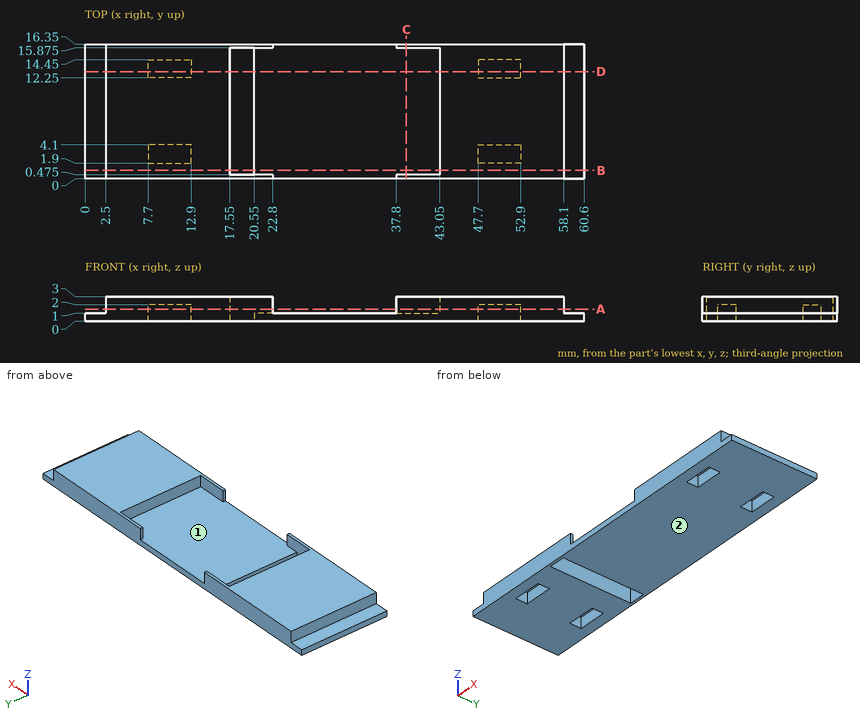
Part print with two shaded views. Sizes in mm from the minimum x, y, z corner. Round coordinates to 2 decimals unless told otherwise and drop trailing zeros. Order: outer loops, then holes, each group sorted by start corner. A loop starts at its lowest first (then second) coordinate and runs counter-clockwise, first axis right, second up. Notation, with made-up numbers: (9, 24) -> (29, 24) arc R16 ccw to (29, 53) -> close; hole circle Ø1 at (36, -22.5). An arc over 180 degrees is marked (long way). Use one line per item in the form item = value.
Item 1: Cut at B-B, the plane y = 1. Write the cut outline in (x, z), and give its area (3 significant figures).
Returned:
outline = (0, 0) -> (17.55, 0) -> (17.55, 3) -> (2.5, 3) -> (2.5, 1) -> (0, 1) -> close; (20.55, 0) -> (60.6, 0) -> (60.6, 1) -> (58.1, 1) -> (58.1, 3) -> (43.05, 3) -> (43.05, 1) -> (20.55, 1) -> close
area = 118 mm^2
Item 2: Cut at A-A, the plane z = 1.5. Give the number of separate pieces and of enclosed holes in the cut face, and give its area (3 significant figures).
Returned:
separate_pieces = 2
enclosed_holes = 4
area = 456 mm^2
Item 3: Pull direction X, two halves, no side cores. Call the marked faces 1 and 2: released by +X, released by -X, zero draft, split by the parting line, or undercut.
Returned:
face_1 = undercut
face_2 = zero draft
Item 4: Cut at C-C, the plane x = 39. Write the cut outline in (y, z) (3 decimals).
Returned:
outline = (0, 0) -> (16.35, 0) -> (16.35, 3) -> (15.875, 3) -> (15.875, 1) -> (0.475, 1) -> (0.475, 3) -> (0, 3) -> close
Item 5: Cut at D-D, the plane y = 13. Write the cut outline in (x, z).
Returned:
outline = (0, 0) -> (7.7, 0) -> (7.7, 2) -> (12.9, 2) -> (12.9, 0) -> (17.55, 0) -> (17.55, 3) -> (2.5, 3) -> (2.5, 1) -> (0, 1) -> close; (20.55, 0) -> (47.7, 0) -> (47.7, 2) -> (52.9, 2) -> (52.9, 0) -> (60.6, 0) -> (60.6, 1) -> (58.1, 1) -> (58.1, 3) -> (43.05, 3) -> (43.05, 1) -> (20.55, 1) -> close
Item 6: Drill centre lines: line 1 (X direction, y = 14.25, z = 0.7); line 2 (Y direction, x = 48, z = 0.95); line 3 (X direction, y = 12.5, z = 2.6). Where is each one in solid material? Low to high.
Returned:
line_1 = 0 to 7.7, 12.9 to 17.55, 20.55 to 47.7, 52.9 to 60.6
line_2 = 0 to 1.9, 4.1 to 12.25, 14.45 to 16.35
line_3 = 2.5 to 17.55, 43.05 to 58.1
Item 7: Flat gauge pins, fed straight in: pin 1 Ø1.8 at (x, y) = (50, 13.5) entering from -Z; pin 2 Ø0.5 at (y, z) = (0.5, 1.5) entering from -X; pin 3 Ø1.5 at (y, z) = (4.5, 2) entering from +X. Where does each tip first touch, or does it go through?
Returned:
pin_1 = 2
pin_2 = 2.5
pin_3 = 58.1
